Geometry: see drawing. Coordinates: mm, zero at the bounding-box minimum. A direction names the side the tool comes from. Give positions to 0.01 mm unless a question says otherwise; leave off trailing zeros. Loops run counter-clockwise (first coordinate to the right, second up) from the corner with the lowest first, then second, coordinate; pieces in that order, holes last. Notation, with made-up numbers: M -13,30.5 L 33,30.5 A18 ccw 33,44.5 Z; hole C 31.5,67.5 d1. An arc over 180 degrees is marked long. Put each result on its own line as item: value.
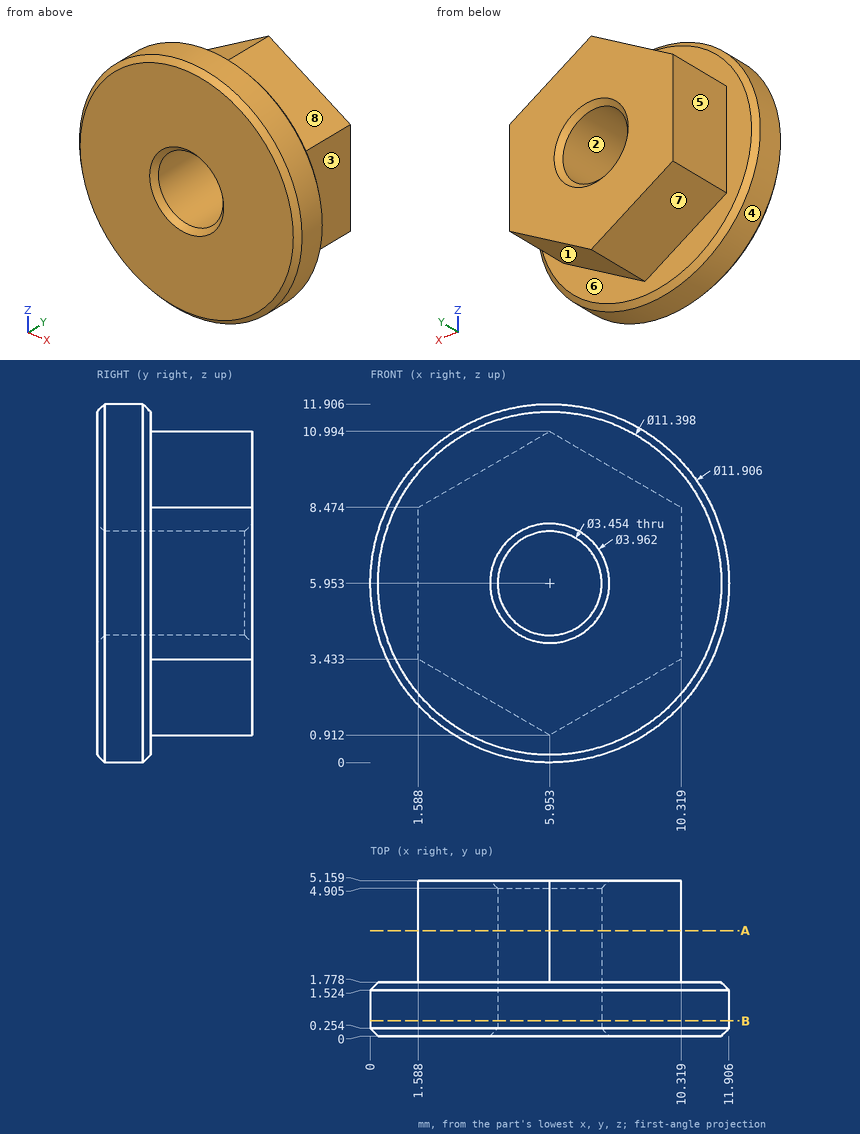
Item 1: Section B-B on y = 0.5. Output: boundary loops of the cut face in (x, z) (1 decimal).
Output values:
outline: C 6,6 d11.9; hole C 6,6 d3.5
Item 2: Mould query, pull axis Z, two halves, no side actions, for the marked faces 1, 2, 3 and 4. Classes: pulls with the +Z half, pulls with the -Z half, needs draft (parallel to the pull), parting line crosses it, or undercut.
Output values:
face 1: pulls with the -Z half
face 2: undercut
face 3: needs draft
face 4: parting line crosses it
Item 3: Section A-A on y = 3.5. Output: boundary loops of the cut face in (x, z) (1 decimal).
Output values:
outline: M 1.6,3.4 L 6,0.9 L 10.3,3.4 L 10.3,8.5 L 6,11 L 1.6,8.5 Z; hole C 6,6 d3.5
Item 4: Line query: probe 1 along Y at (x, z) = (2.5, 10); probe 2 along Z at (x, y) = (6.5, 2.5) (1 decimal); probe 3 along X at (y, z) = (4.8, 7) (1 decimal). Output: solid intervals per line, ascending. Write a range as [from, to].
Output values:
probe 1: [0, 1.78]
probe 2: [1.2, 4.3], [7.6, 10.7]
probe 3: [1.6, 4.6], [7.3, 10.3]
Item 5: Set-up query: the marked faces 5, 6, 7 and 8. Return all of +Z, -Z, +X, -X, +Y, -Y with unobstructed straight access to the full face (end or side cutting, diameter ignored); none if empty.
Output values:
face 5: +Z, -Z, -X, +Y
face 6: +Y
face 7: -Z, -X, +Y
face 8: +Z, +X, +Y
Item 6: Pin query (flat end, axial travel): pin 1 Ø3 at (x, y) = (2, 2.5) entering from -Z; pin 2 Ø3 at (x, z) = (5.95, 5.95) entering from +Y; pin 3 Ø3 at (y, z) = (4, 4) entering from +X; pin 4 Ø1 at (x, y) = (5.5, 4) entering from +Z. Return the tip coordinate at first contact, or that it passes through.
Output values:
pin 1: z = 0.71
pin 2: through
pin 3: x = 10.32
pin 4: z = 10.99
